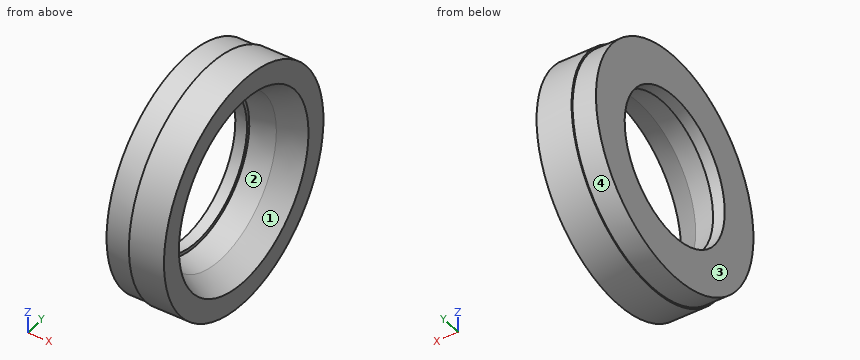
from build123d import *

# Parameters (mm, degrees)
F2_W = 8
F2_H = 0.5


with BuildPart() as f1:
    # F0 (on Front) → F1 (revolve)
    with BuildSketch(Plane.XZ):
        Polygon((20, 40), (0, 40), (0, 25.1), (4, 25.1), (4, 26.25), (12, 28.0972), (20, 32.5), align=None)
    revolve(axis=Axis((11.28888, 0, 0), (1, 0, 0)))

    # F2 (on Front) → F3 (revolve, cut)
    with BuildSketch(Plane.XZ):
        with Locations((4, 39.75)):
            Rectangle(F2_W, F2_H)
    revolve(axis=Axis((17.787712, 0, 0), (1, 0, 0)), mode=Mode.SUBTRACT)


solid = f1.part
Model file for the job. Use its own axes, mm. Face numbers are marked on the shaded views. Coordinates: 2 decimals unless noted, no trailing zeros. Order: outer loops, then holes, each group sorted by start corner. A loop starts at its lowest first (then second) coordinate and runs counter-clockwise, first axis right, second up. Notation, with made-up numbers: (5, 14.5) -> (56, 14.5) arc R18 cw to (56, 43.5) -> close; hole circle Ø8 at (23.5, 51). An arc over 180 degrees is marked (long way). Return JSON: item names as keys, results as strings. Group by question number.
Item 1: Saw through at A-A on z = 0. Write the cut outline in (x, y), then the cut area to 3 significant figures.
Item 2: Pull direction Y, two halves, no side cores. Call the marked faces 1, 2, 3 and 4: pulls with the +Y half, pulls with the -Y half, needs draft (parallel to the pull), parting line crosses it, or undercut.
Item 3: Wall check: line 1 along Y through (x, z) = (2.8, 0); line 2 along Y through (x, z) = (1.5, -15.5). Give the ranges that are in metal, low to high. Write a range as [from, to].
Item 4: Saw through at D-D on x = 14. Write the cut outline in (y, z), then the cut area to 3 significant figures.
Item 5: Flat gauge pins, fed straight in: P1, Ø2, axis at x = 15, y = 2.5, coming from the +Z side; P2, Ø2, axis at x = 10, z = -27.5, coming from the -Y side; P3, Ø5, axis at x = 14.5, z = -20.5, coming from the +Y side. Where does each tip first touch, or does it go through?
Item 6: Saw through at C-C on x = 9. Write the cut outline in (y, z), then the cut area to 3 significant figures.
Values found:
{
 "1": {"outline": "(0, -39.5) -> (8, -39.5) -> (8, -40) -> (20, -40) -> (20, -32.5) -> (12, -28.1) -> (4, -26.25) -> (4, -25.1) -> (0, -25.1) -> close; (0, 25.1) -> (4, 25.1) -> (4, 26.25) -> (12, 28.1) -> (20, 32.5) -> (20, 40) -> (8, 40) -> (8, 39.5) -> (0, 39.5) -> close", "area": "472 mm2"},
 "2": {"face 1": "undercut", "face 2": "undercut", "face 3": "needs draft", "face 4": "parting line crosses it"},
 "3": {"line 1": "y = [-39.5, -25.1], [25.1, 39.5]", "line 2": "y = [-36.33, -19.74], [19.74, 36.33]"},
 "4": {"outline": "circle Ø80 at (0, 0); hole circle Ø58.4 at (0, 0)", "area": "2,350 mm2"},
 "5": {"P1": "stops at z = 39.97", "P2": "stops at y = -29.96", "P3": "stops at y = 35.72"},
 "6": {"outline": "circle Ø80 at (0, 0); hole circle Ø54.81 at (0, 0)", "area": "2,670 mm2"}
}
